```python
from build123d import *

# Parameters (mm, degrees)
FILLET1_R          = 0.762
FILLET2_R          = 0.762
CUT_EXTRUDE2_START = -17.8562
SKETCH2_R          = 3.96875
CUT_EXTRUDE2_DEPTH = 35.7124
CUT_EXTRUDE4_START = 17.8562
SKETCH3_R          = 5.1562
CUT_EXTRUDE4_DEPTH = 35.7124
CUT_EXTRUDE6_START = 17.8562
SKETCH4_R          = 7.9375
CUT_EXTRUDE6_DEPTH = 9.525


with BuildPart() as part:
    # Sketch1 → Revolve1 (revolve)
    with BuildSketch(Plane(origin=(0, 0, 0), x_dir=(1, 0, 0), z_dir=(0, 1, 0)), mode=Mode.PRIVATE) as revolve1_sk:
        Polygon((-17.8562, 253.9111), (-2.6162, 253.9111), (-2.6162, 234.188), (17.8562, 234.188), (17.8562, 196.85), (-2.6162, 196.85), (-2.6162, 215.9127), (-17.8562, 215.9127), align=None)
    revolve(revolve1_sk.sketch.rotate(Axis((-43.2562, 0, 0), (1, 0, 0)), 180), axis=Axis((-43.2562, 0, 0), (1, 0, 0)))

    # Fillet1
    fillet1_edges = [part.edges().sort_by_distance(p)[0] for p in [
        (-2.6162, 0, -234.188),
    ]]
    fillet(fillet1_edges, radius=FILLET1_R)

    # Fillet2
    fillet2_edges = [part.edges().sort_by_distance(p)[0] for p in [
        (-2.6162, 0, -215.9127),
    ]]
    fillet(fillet2_edges, radius=FILLET2_R)

    # Sketch2 → Cut-Extrude2 (cut)
    with BuildSketch(Plane(origin=(0, 0, 0), x_dir=(0, 0, -1), z_dir=(1, 0, 0)).offset(CUT_EXTRUDE2_START)):
        with Locations(Location((244.475, 0, 0), (0, 0, 180))):
            Circle(SKETCH2_R)
        with Locations(Location((172.8699362, 172.8699362, 0), (0, 0, 180))):
            Circle(SKETCH2_R)
        with Locations(Location((0, 244.475, 0), (0, 0, 180))):
            Circle(SKETCH2_R)
        with Locations(Location((-172.8699362, 172.8699362, 0), (0, 0, 180))):
            Circle(SKETCH2_R)
        with Locations(Location((-244.475, 0, 0), (0, 0, 180))):
            Circle(SKETCH2_R)
        with Locations(Location((-172.8699362, -172.8699362, 0), (0, 0, 180))):
            Circle(SKETCH2_R)
        with Locations(Location((0, -244.475, 0), (0, 0, 180))):
            Circle(SKETCH2_R)
        with Locations(Location((172.8699362, -172.8699362, 0), (0, 0, 180))):
            Circle(SKETCH2_R)
    extrude(amount=CUT_EXTRUDE2_DEPTH, mode=Mode.SUBTRACT)

    # Sketch3 → Cut-Extrude4 (cut)
    with BuildSketch(Plane(origin=(0, 0, 0), x_dir=(0, 0, -1), z_dir=(1, 0, 0)).offset(CUT_EXTRUDE4_START)):
        with Locations((206.375, 0)):
            Circle(SKETCH3_R)
        with Locations((145.9291722, 145.9291722)):
            Circle(SKETCH3_R)
        with Locations((0, 206.375)):
            Circle(SKETCH3_R)
        with Locations((-145.9291722, 145.9291722)):
            Circle(SKETCH3_R)
        with Locations((-206.375, 0)):
            Circle(SKETCH3_R)
        with Locations((-145.9291722, -145.9291722)):
            Circle(SKETCH3_R)
        with Locations((0, -206.375)):
            Circle(SKETCH3_R)
        with Locations((145.9291722, -145.9291722)):
            Circle(SKETCH3_R)
    extrude(amount=-CUT_EXTRUDE4_DEPTH, mode=Mode.SUBTRACT)

    # Sketch4 → Cut-Extrude6 (cut)
    with BuildSketch(Plane(origin=(0, 0, 0), x_dir=(0, 0, -1), z_dir=(1, 0, 0)).offset(CUT_EXTRUDE6_START)):
        with Locations((206.375, 0)):
            Circle(SKETCH4_R)
        with Locations((145.9291722, 145.9291722)):
            Circle(SKETCH4_R)
        with Locations((0, 206.375)):
            Circle(SKETCH4_R)
        with Locations((-145.9291722, 145.9291722)):
            Circle(SKETCH4_R)
        with Locations((-206.375, 0)):
            Circle(SKETCH4_R)
        with Locations((-145.9291722, -145.9291722)):
            Circle(SKETCH4_R)
        with Locations((0, -206.375)):
            Circle(SKETCH4_R)
        with Locations((145.9291722, -145.9291722)):
            Circle(SKETCH4_R)
    extrude(amount=-CUT_EXTRUDE6_DEPTH, mode=Mode.SUBTRACT)


solid = part.part
```
Could you check a few things on this model? Use its own coordinates, in mm. A direction names the side the tool comes from. Give positions to 0.01 mm unless a question says otherwise; leave off trailing zeros. Put each result on its own line as item: value.
(1) Please list where these lines run through material, in increasing order: probe 1 along X at (y, z) = (181.5, -113.5); probe 2 along Y at (x, z) = (-7, -197); probe 3 along Z at (x, y) = (-10.5, 43). Write a range as [from, to].
Computed:
probe 1: [-2.62, 17.86]
probe 2: [-160.19, -88.37], [88.37, 160.19]
probe 3: [-250.24, -211.59], [211.59, 250.24]
(2) I'm going to push flat-ended pins straight in: pin 1 Ø6 at (x, y) = (8.5, 134.5) entering from -Z; pin 2 Ø9.5 at (y, z) = (-145.93, -145.93) entering from -X (3 decimals); pin 3 Ø2 at (x, z) = (-2.5, -144.5) entering from -Y; pin 4 Ø12.5 at (y, z) = (-145.93, 145.93) entering from -X. Where does each tip first touch, or does it pass through?
Computed:
pin 1: z = -193.78
pin 2: through
pin 3: y = -209.47
pin 4: x = -2.62
(3) For faces 1 (the face through (-10.13, -76.268, 242.186)), 2 (the face through (8.331, 140.7, 144.3)), which set-ups out of +Z, -Z, +X, -X, +Y, -Y let a thin tool reach every point of the face, with its end or its side?
Computed:
face 1: +X, -X
face 2: +X
(4) Thinking about a two-plate mould opening in Y: for faces 3 (the face through (8.139, -158.275, -172.606)), 4 (the face through (13.16, -199.682, -4.267)), 5 (the face through (17.856, -140, -140)), which applies, pulls with the +Y half, pulls with the -Y half, needs draft (parallel to the pull), parting line crosses it, or undercut?
Computed:
face 3: parting line crosses it
face 4: undercut
face 5: needs draft
